The listing builds one solid part. Answer for the finished solid, in the listing's coordinates (mm). A direction names the side the tool comes from. Give positions to 0.01 mm unless a question says otherwise; leave off trailing zeros. Write each loop counter-clockwise with the first axis right and the second up, starting at its lowest first coordinate (ties: lowest second). Pieces come first, ordered by that corner, then holes. Notation, with made-up numbers: M 14.25,-3.75 L 39.25,-3.75 A25 cw 39.25,9.25 Z; hole C 57,54 d11. An arc over 180 degrees is marked long. Answer as a JSON object with one key per item and string values.
```python
from build123d import *

# Parameters (mm, degrees)
SKETCH1_W           = 241.3
SKETCH1_H           = 76.2
SKETCH1_W_2         = 205.74
SKETCH1_H_2         = 5.588
BOSS_EXTRUDE1_DEPTH = 149.86
SHELL1_START        = -117.475
SHELL1_OUTLINE_W    = 149.86
SHELL1_OUTLINE_H    = 69.85
SHELL1_DEPTH        = 234.95
CUT_EXTRUDE1_START  = -76.2
CUT_EXTRUDE1_DEPTH  = 3.175


# Read off the part's stored shape, not the designer's step: Shell1
with BuildPart() as part:
    # Sketch1 → Boss-Extrude1 (new body)
    with BuildSketch(Plane(origin=(0, 0, 0), x_dir=(1, 0, 0), z_dir=(0, 1, 0))):
        Rectangle(SKETCH1_W, SKETCH1_H)
        Rectangle(SKETCH1_W_2, SKETCH1_H_2, mode=Mode.SUBTRACT)
    extrude(amount=BOSS_EXTRUDE1_DEPTH)

    # Shell1 outline → Shell1 (cut)
    with BuildSketch(Plane.YZ.offset(SHELL1_START)):
        with Locations((74.93, 0)):
            Rectangle(SHELL1_OUTLINE_W, SHELL1_OUTLINE_H)
    extrude(amount=SHELL1_DEPTH, mode=Mode.SUBTRACT)

    # Sketch3 → Cut-Extrude1 (cut)
    with BuildSketch(Plane.XY.offset(38.1).offset(CUT_EXTRUDE1_START)):
        Polygon((107.95, 52.944691481), (66.675, 28.786196813), (107.95, 14.844691481), align=None)
        Polygon((98.425, 12.7), (60.325, 25.569081846), (22.225, 12.7), align=None)
        Polygon((97.597199346, 52.771327471), (60.325, 30.955695027), (23.052800654, 52.771327471), align=None)
        Polygon((53.975, 28.786196813), (12.7, 14.844691481), (12.7, 52.944691481), align=None)
        Polygon((-107.95, 52.944691481), (-66.675, 28.786196813), (-107.95, 14.844691481), align=None)
        Polygon((-22.225, 12.7), (-60.325, 25.569081846), (-98.425, 12.7), align=None)
        Polygon((-12.7, 52.944691481), (-53.975, 28.786196813), (-12.7, 14.844691481), align=None)
        Polygon((-97.597199346, 52.771327471), (-60.325, 30.955695027), (-23.052800654, 52.771327471), align=None)
    extrude(amount=CUT_EXTRUDE1_DEPTH, mode=Mode.SUBTRACT)


solid = part.part
```
1. For faces 4 (the flat face through (117.475, 74, 0)), 5 (the flat face through (-33.049, 41.035, -36.535)), 6 (the flat face through (-2, 74, 38.1)), determine the directions among +Z, -Z, +X, -X, +Y, -Y from which every point of the face is accessible in a straight line to the end or side of a thin tool.
Verdict:
{"face 4": "+Y, -Y", "face 5": "-Z", "face 6": "+Z, +X, -X, +Y, -Y"}
2. A cutting plane is placed at A-A, the plane x = -9.5. Give the vertices of the cut face in (y, z) (3 decimals).
Verdict:
{"outline": "M 0,-38.1 L 149.86,-38.1 L 149.86,-34.925 L 0,-34.925 Z; M 0,34.925 L 149.86,34.925 L 149.86,38.1 L 0,38.1 Z"}
3. The mould has two halves that part along Y. Classify faces 1 (the flat face through (-120.65, 74, 1)), 2 (the flat face through (-1, 0, -37)), 3 (the flat face through (-79.222, 42.016, -36.535)): released by +Y, released by -Y, zero draft, split by the parting line, or undercut.
Verdict:
{"face 1": "zero draft", "face 2": "released by -Y", "face 3": "undercut"}
4. A cutting plane is placed at B-B, the plane y = 76.5. Give the vertices of the cut face in (x, z) (3 decimals), plus the area to 3 significant figures.
Verdict:
{"outline": "M -120.65,-38.1 L 120.65,-38.1 L 120.65,38.1 L -120.65,38.1 Z; hole M -117.475,-34.925 L 117.475,-34.925 L 117.475,34.925 L -117.475,34.925 Z", "area": "1,980 mm2"}
5. Consider line 1 along X through (y, z) = (116, 8) (3 decimals); line 2 along Z through (x, y) = (-12.5, 104.5) (3 decimals); line 3 along Y through (x, z) = (35.5, -35). Determine where each line is inside the solid, lowest interval first.
Verdict:
{"line 1": "x = -120.65 to -117.475, 117.475 to 120.65", "line 2": "z = -38.1 to -34.925, 34.925 to 38.1", "line 3": "y = 0 to 12.7, 17.18 to 22.55, 39.6 to 45.49, 52.77 to 149.86"}
6. A cutting plane is placed at C-C, the plane z = 25. Give the vertices of the cut face in (x, y) (3 decimals).
Verdict:
{"outline": "M -120.65,0 L -117.475,0 L -117.475,149.86 L -120.65,149.86 Z; M 117.475,0 L 120.65,0 L 120.65,149.86 L 117.475,149.86 Z"}
7. A cutting plane is placed at D-D, the plane x = -94. Give the vertices of the cut face in (y, z) (3 decimals).
Verdict:
{"outline": "M 0,-38.1 L 12.7,-38.1 L 12.7,-34.925 L 0,-34.925 Z; M 0,34.925 L 149.86,34.925 L 149.86,38.1 L 0,38.1 Z; M 14.195,-38.1 L 19.557,-38.1 L 19.557,-34.925 L 14.195,-34.925 Z; M 44.78,-38.1 L 50.666,-38.1 L 50.666,-34.925 L 44.78,-34.925 Z; M 52.771,-38.1 L 149.86,-38.1 L 149.86,-34.925 L 52.771,-34.925 Z"}
